Could you check a few things on this drawing? It's one solid part, dimensions in mm from its lowest x, y, z. A direction names the side the tool comes from. Give positions to 0.01 mm unless a question says otherwise; leave off trailing zeros. Loops run counter-clockwise (first coordinate to the right, second up) from the corner with the lowest first, then second, coordinate; pieces in that order, holes last.
1. Imagine slicing it at B-B (y = 40.5). List the corners of the cut face in (x, z) for me.
2. For P1, Ø5, axis at x = 10.5, y = 54.5, coming from the +Z side; P2, Ø12, axis at x = 49.5, z = 70, coming from the -Y side, each with a flat end and sliding along its axis, tell me the tip position at first contact or that it passes through.
3. For the marked faces 1 and 2, which set-ups out of +Z, -Z, +X, -X, +Y, -Y let a thin tool reach every point of the face, with its end or its side?
4. I need wall thicknesses on line 1 along Z through (x, y) = (35, 48); line 2 along Y through (x, z) = (35.5, 67) (1 decimal); line 3 along Y through (x, z) = (37.5, 77) (1 decimal). Which ranges of each line are inside material? Lowest first, please.
5. Imagine slicing it at C-C (z = 76.5). List the corners of the cut face in (x, y) for me (1 decimal).
6. Imagine slicing it at A-A (x = 39). List the corners of the cut face in (y, z) for me (1 decimal).
7. Imagine slicing it at D-D (y = 65). List the corners of the cut face in (x, z) for me, plus the area to 3 significant figures.
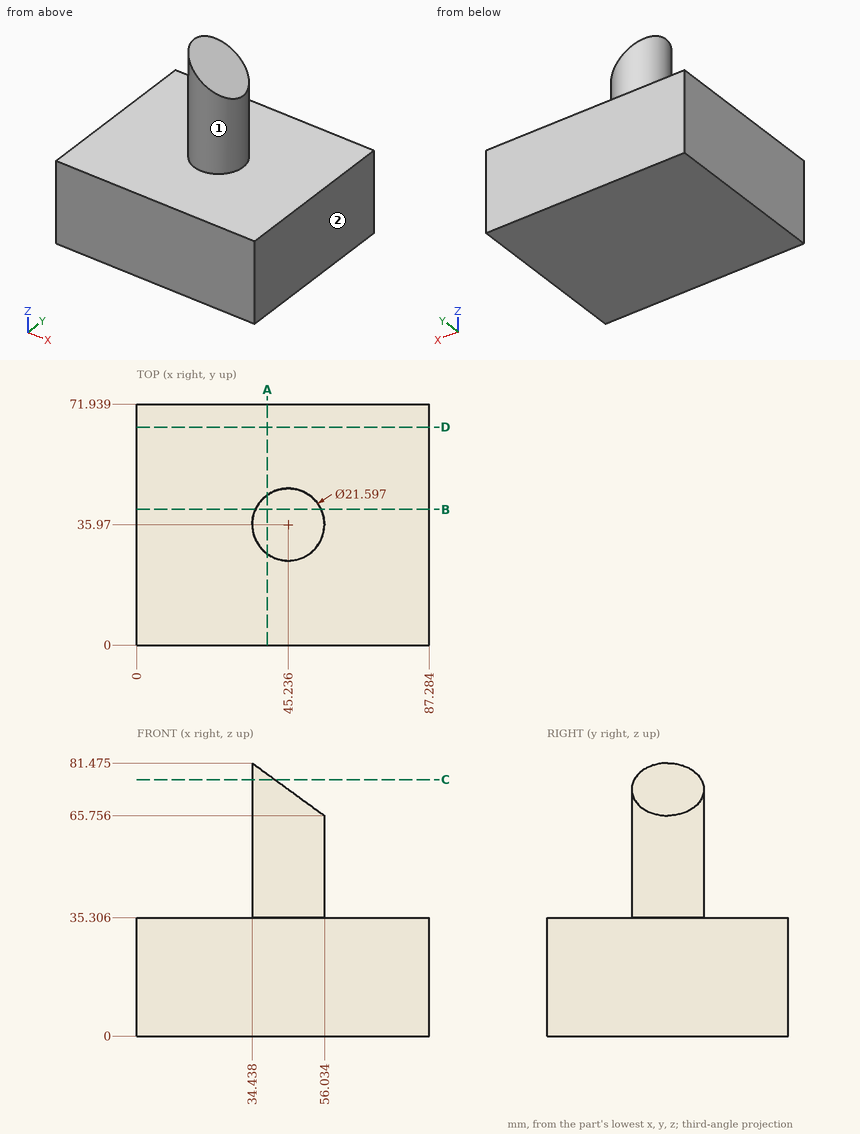
Derived:
1. outline: (0, 0) - (87.28, 0) - (87.28, 35.31) - (55.04, 35.31) - (55.04, 66.48) - (35.43, 80.75) - (35.43, 35.31) - (0, 35.31) - close
2. P1: stops at z = 35.31
2. P2: stops at y = 25.17
3. face 1: +Z
3. face 2: +Z, -Z, +X, +Y, -Y
4. line 1: z = 0 to 35.31
4. line 2: y = 31.3 to 40.6
4. line 3: y = 28.4 to 43.5
5. outline: (41.3, 25.9) - (41.3, 46) arc R10.8 ccw to start
6. outline: (0, 0) - (71.9, 0) - (71.9, 35.3) - (44.8, 35.3) - (44.8, 78.2) - (27.2, 78.2) - (27.2, 35.3) - (0, 35.3) - close
7. outline: (0, 0) - (87.28, 0) - (87.28, 35.31) - (0, 35.31) - close
7. area: 3,080 mm2
